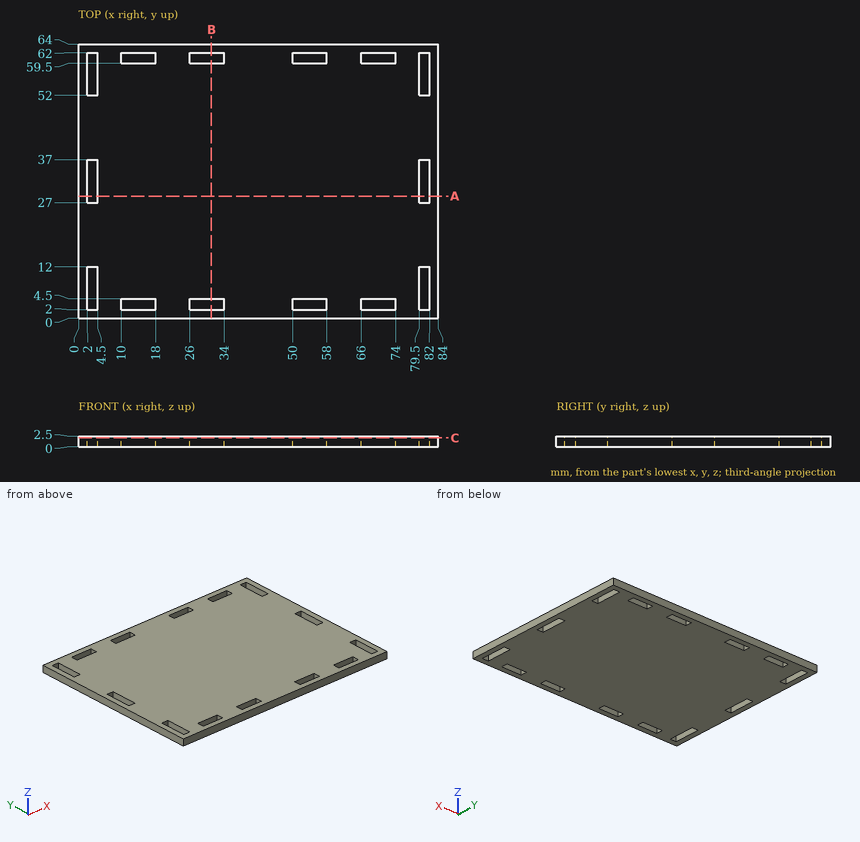
Could you check a few things on this drawing? It's one solid part, dimensions in mm from its lowest x, y, z. Give positions to 0.01 mm unless a question says otherwise; leave off trailing zeros. Order: outer loops, then holes, each group sorted by start corner. A loop starts at its lowest first (then second) coordinate and runs counter-clockwise, first axis right, second up.
1. Suppose I cut it at B-B (x = 31). Write out the boundary of the cut face in (y, z).
Answers below:
outline: (0, 0) - (2, 0) - (2, 2.5) - (0, 2.5) - close; (4.5, 0) - (59.5, 0) - (59.5, 2.5) - (4.5, 2.5) - close; (62, 0) - (64, 0) - (64, 2.5) - (62, 2.5) - close
2. I need wall thicknesses on L1, parallel to X at y = 32, z = 1.1; L2, parallel to Y at x = 12, z = 1.8; L3, parallel to Y at x = 80.5, z = 0.6. Which ranges of each line are inside material? Lowest first, please.
Answers below:
L1: x = 0 to 2, 4.5 to 79.5, 82 to 84
L2: y = 0 to 2, 4.5 to 59.5, 62 to 64
L3: y = 0 to 2, 12 to 27, 37 to 52, 62 to 64
3. Suppose I cut it at C-C (z = 2.1). State how many separate pieces and enclosed holes the cut face has, plus the area to 3 significant figures.
Answers below:
separate pieces: 1
enclosed holes: 14
area: 5,070 mm2
4. Suppose I cut it at A-A (y = 28.5). Write out the boundary of the cut face in (x, z).
Answers below:
outline: (0, 0) - (2, 0) - (2, 2.5) - (0, 2.5) - close; (4.5, 0) - (79.5, 0) - (79.5, 2.5) - (4.5, 2.5) - close; (82, 0) - (84, 0) - (84, 2.5) - (82, 2.5) - close
